Design review of the part built by this model. Coordinates are the model's own, in mm. Face numbers are marked on the shaded views. Round coordinates to 2 decimals unless told otherwise and drop trailing zeros. Loops run counter-clockwise (first coordinate to the right, second up) from the corner with the lowest first, then second, coordinate; pieces in that order, holes last. Notation, with made-up numbers: (42.25, -33) - (82.25, -33) arc R24 cw to (82.25, -16) - close; hole circle Ø7 at (-2.5, -13). An arc over 180 degrees is marked (long way). Use one line per item in the form item = value. Start each with the question number.
(1) We need section A-A, the plane x = 0. Write out the cut boundary in (y, z), then the cut area to 3 significant figures.
(2) We need section C-C, the plane y = 2.75. Write out the cut boundary in (x, z), then the cut area to 3 significant figures.
(3) We need section D-D, the plane y = -5.25. Write out the cut boundary in (x, z).
(4) The part is to be moulded in two halves that separate along Y. For the marked faces 1, 2, 3 and 4, say which applies: released by +Y, released by -Y, zero draft, split by the parting line, or undercut.
(5) Wall thickness on probe 1 along Y at (x, z) = (1, -29.5); probe 2 along Y at (x, z) = (0, 0.6); probe 3 along X at (y, z) = (0, -14.5): over which ranges is each line inside the solid? List them lowest first. Write a range as [from, to].
(6) For pin 1 (5 mm diameter, centred on x = 0, y = 0, fed in from +Z); pin 2 (12 mm diameter, centred on x = 9.5, z = -5, fed in from +Y); pin 3 (4 mm diameter, centred on y = 1, z = -34.5, fed in from +X); pin 4 (3 mm diameter, centred on y = 5, z = -35.5, fed in from -X), all flat-tipped, find the tip position at first contact; note any pin that passes through.
Autodesk Inventor part; units mm, degrees
ref_plane "YZ Plane" through (0, 0, 0) normal (1, 0, 0) x (0, 1, 0)
ref_plane "XZ Plane" through (0, 0, 0) normal (0, 1, 0) x (-1, 0, 0)
ref_plane "XY Plane" through (0, 0, 0) normal (0, 0, 1) x (1, 0, 0)
sketch "Sketch1" plane through (0, 0, 0) normal (0, 0, 1) x (1, 0, 0)
  line L0 (5.4993, 3.175) -> (7.3323, 0)
  line L1 (0, 6.35) -> (3.6662, 6.35)
  line L2 (3.6662, 6.35) -> (5.4993, 3.175)
  line L3 (7.3323, 0) -> (5.4993, -3.175)
  line L4 (5.4993, -3.175) -> (3.6662, -6.35)
  line L5 (3.6662, -6.35) -> (0, -6.35)
  line L6 (0, -6.35) -> (-3.6662, -6.35)
  line L7 (-3.6662, -6.35) -> (-5.4993, -3.175)
  line L8 (-5.4993, -3.175) -> (-7.3323, 0)
  line L9 (-7.3323, 0) -> (-5.4993, 3.175)
  line L10 (-5.4993, 3.175) -> (-3.6662, 6.35)
  line L11 (-3.6662, 6.35) -> (0, 6.35)
  line L12 (5.6725, 3.275) -> (7.5633, 0)
  line L13 (7.5633, 0) -> (5.6725, -3.275)
  line L14 (5.6725, -3.275) -> (3.7816, -6.55)
  line L15 (3.7816, -6.55) -> (0, -6.55)
  line L16 (0, -6.55) -> (-3.7816, -6.55)
  line L17 (-3.7816, -6.55) -> (-5.6725, -3.275)
  line L18 (-5.6725, -3.275) -> (-7.5633, 0)
  line L19 (-7.5633, 0) -> (-5.6725, 3.275)
  line L20 (-5.6725, 3.275) -> (-3.7816, 6.55)
  line L21 (-3.7816, 6.55) -> (0, 6.55)
  line L22 (0, 6.55) -> (3.7816, 6.55)
  line L23 (3.7816, 6.55) -> (5.6725, 3.275)
  line L24 (10.0026, 5.775) -> (13.3368, 0)
  line L25 (13.3368, 0) -> (10.0026, -5.775)
  line L26 (10.0026, -5.775) -> (6.6684, -11.55)
  line L27 (6.6684, -11.55) -> (0, -11.55)
  line L28 (0, -11.55) -> (-6.6684, -11.55)
  line L29 (-6.6684, -11.55) -> (-10.0026, -5.775)
  line L30 (-10.0026, -5.775) -> (-13.3368, 0)
  line L31 (-13.3368, 0) -> (-10.0026, 5.775)
  line L32 (-10.0026, 5.775) -> (-6.6684, 11.55)
  line L33 (-6.6684, 11.55) -> (0, 11.55)
  line L34 (0, 11.55) -> (6.6684, 11.55)
  line L35 (6.6684, 11.55) -> (10.0026, 5.775)
  point P0 (0, 0)
  dimension "d0" = 0.2
  dimension "d1" = 5
extrude "Extrusion1" add sketch "Sketch1" against normal blind 40 contours L24 L25 L26 L27 L28 L29 L30 L31 L32 L33 L34 L35
sketch "Sketch2" plane through (0, 0, 0) normal (0, 0, 1) x (1, 0, 0)
  line L0 (-3.7816, 6.55) -> (3.7816, 6.55)
  line L1 (3.7816, 6.55) -> (7.5633, 0)
  line L2 (7.5633, 0) -> (3.7816, -6.55)
  line L3 (3.7816, -6.55) -> (-3.7816, -6.55)
  line L4 (-3.7816, -6.55) -> (-7.5633, 0)
  line L5 (-7.5633, 0) -> (-3.7816, 6.55)
  line L6 (6.6684, 11.55) -> (13.3368, 0)
  line L7 (-6.6684, 11.55) -> (6.6684, 11.55)
  line L8 (-13.3368, 0) -> (-6.6684, 11.55)
  line L9 (-6.6684, -11.55) -> (-13.3368, 0)
  line L10 (6.6684, -11.55) -> (-6.6684, -11.55)
  line L11 (13.3368, 0) -> (6.6684, -11.55)
  point P0 (0, 0)
extrude "Extrusion2" add sketch "Sketch2" along normal blind 2 contours L0 L1 L2 L3 L4 L5 | L6 L11 L10 L9 L8 L7
sketch "Sketch3" plane through (0, 0, 2) normal (0, 0, 1) x (1, 0, 0)
  point P0 (0, 0)
  point P1 (0, 0)
hole "Hole1" at (0, 0, 2) direction (0, 0, -1) diameter 8.4375 end through all
properties part number "AntiBacklash" material "ABS Plastic"
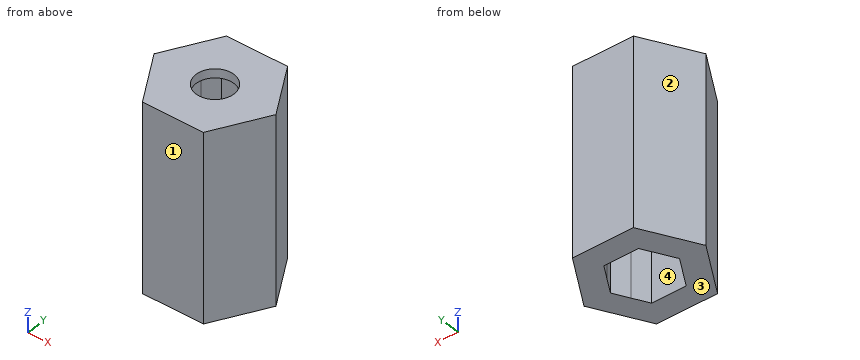
Data:
q1.outline = (-11.55, -40) - (-6.55, -40) - (-6.55, 0) - (-4.22, 0) - (-4.22, 2) - (-11.55, 2) - close; (4.22, 0) - (6.55, 0) - (6.55, -40) - (11.55, -40) - (11.55, 2) - (4.22, 2) - close
q1.area = 429 mm^2
q2.outline = (-11.75, -40) - (-5.98, -40) - (-5.98, 0) - (-3.2, 0) - (-3.2, 2) - (-11.75, 2) - close; (3.2, 0) - (5.98, 0) - (5.98, -40) - (11.75, -40) - (11.75, 2) - (3.2, 2) - close
q2.area = 496 mm^2
q3.outline = (-10.31, -40) - (-4.53, -40) - (-4.53, 0) - (4.53, 0) - (4.53, -40) - (10.31, -40) - (10.31, 2) - (-10.31, 2) - close
q4.face_1 = released by -Y
q4.face_2 = released by +Y
q4.face_3 = zero draft
q4.face_4 = undercut
q5.probe_1 = [-11.55, -6.55], [6.55, 11.55]
q5.probe_2 = [-11.55, -4.22], [4.22, 11.55]
q5.probe_3 = [-13.34, -7.56], [7.56, 13.34]
q6.pin_1 = through
q6.pin_2 = 11.55
q6.pin_3 = 13.34
q6.pin_4 = -11.32
